Design review of the part built by this model. Coordinates are the model's own, in mm. A direction names the side the tool comes from. Round coordinates to 2 decimals unless told otherwise and drop trailing zeros. Order: outer loops, then holes, each group sorted by start corner. A loop starts at its lowest first (then second) coordinate and runs counter-clockwise, first axis right, second up. Notation, with made-up numbers: (69, -16.5) - (120, -16.5) arc R16 cw to (120, -0.5) - close; hole circle Ø6 at (67.25, 61). An arc over 180 degrees is marked (long way). Answer as a JSON object with one key per item and string values. Group by question number.
from build123d import *

# Parameters (mm, degrees)
F1_DEPTH = 50.8


with BuildPart() as f1:
    # F0 (on Front) → F1 (new body)
    with BuildSketch(Plane.XZ):
        with BuildLine():
            ThreePointArc((-7.481652, 37.285154), (-41.440481, 30.054075), (-70.981652, 11.811))
            Line((-70.981652, 11.811), (-20.181652, 11.811))
            ThreePointArc((-20.181652, 11.811), (-7.481652, 24.455001), (5.218348, 11.811))
            Line((5.218348, 11.811), (81.418348, 11.811))
            ThreePointArc((81.418348, 11.811), (94.118348, 24.369807), (106.818348, 11.811))
            Line((106.818348, 11.811), (157.618348, 11.811))
            ThreePointArc((157.618348, 11.811), (128.077177, 30.054075), (94.118348, 37.285154))
            ThreePointArc((94.118348, 37.285154), (43.318348, 50.896973), (-7.481652, 37.285154))
        make_face()
        with BuildLine():
            ThreePointArc((5.218348, 11.811), (-7.481652, 24.455001), (-20.181652, 11.811))
            ThreePointArc((-20.181652, 11.811), (-7.481652, -0.420556), (5.218348, 11.811))
        make_face()
        with BuildLine():
            ThreePointArc((106.818348, 11.811), (94.118348, 24.369807), (81.418348, 11.811))
            ThreePointArc((81.418348, 11.811), (94.118348, -1.27557), (106.818348, 11.811))
        make_face()
    extrude(amount=F1_DEPTH)


solid = f1.part
1. Tool access review of faces 1 (the flat face through (132, -25, 11.811)), 2 (the flat face through (43, -25, 11.811)), 3 (the flat face through (42, 0, 25)): name each direction out of +Z, -Z, +X, -X, +Y, -Y from which nothing blocks a thin tool from reaching the whole face with its end or side.
2. Take a section at C-C, the plane x = 36. Give the boundary of the cut face in (y, z), then the cut area to 3 significant figures.
3. Clearance check with flat-ended pins moving along their axes: P1, Ø2, axis at y = -10.5, z = 31, coming from the +X side; P2, Ø1, axis at y = -39, z = 21.5, coming from the +X side; P3, Ø2, axis at x = 19.5, y = -32.5, coming from the -Z side. State where each tip first meets the part, or that it passes through.
4. To check wall thickness, follow line 1 (X direction, y = -13.5, z = 11); line 2 (Z direction, x = -17, y = -17); line 3 (Z direction, x = -44.5, y = -7). State the ranges of each line that lie inside material, in increasing order. Write a range as from..to.
5. Take a section at D-D, the plane z = 46. Give the boundary of the cut face in (x, y).
6. Take a section at A-A, the plane z = 9. Give the boundary of the cut face in (x, y), then the cut area to 3 significant figures.
7. Take a section at B-B, the plane y = -9. Give the boundary of the cut face in (x, z), then the cut area to 3 significant figures.
8. Mouldability with a two-part tool opening along X and no side actions: class faces 4 (the cylindrical face through (44.063, -25.044, 50.894)), 5 (the cylindrical face through (93.834, -25.044, -1.272)), 6 (the flat face through (-46, -25, 11.811)) as pulls with the +X half, pulls with the -X half, needs draft (parallel to the pull), parting line crosses it, or undercut.
Response values:
{
 "1": {"face 1": "-Z, +X, +Y, -Y", "face 2": "-Z, +Y, -Y", "face 3": "+Z, -Z, +X, -X, +Y"},
 "2": {"outline": "(-50.8, 11.81) - (0, 11.81) - (0, 50.63) - (-50.8, 50.63) - close", "area": "1,970 mm2"},
 "3": {"P1": "x = 128.21", "P2": "x = 145.53", "P3": "z = 11.81"},
 "4": {"line 1": "-20.13..5.16, 81.42..106.82", "line 2": "3.87..36.47", "line 3": "11.81..28.77"},
 "5": {"outline": "(12.16, -50.8) - (74.48, -50.8) - (74.48, 0) - (12.16, 0) - close"},
 "6": {"outline": "(-19.76, -50.8) - (4.79, -50.8) - (4.79, 0) - (-19.76, 0) - close; (81.65, -50.8) - (106.59, -50.8) - (106.59, 0) - (81.65, 0) - close", "area": "2,510 mm2"},
 "7": {"outline": "(-70.98, 11.81) - (-20.18, 11.81) arc R12.71 ccw to (5.22, 11.81) - (81.42, 11.81) arc R12.71 ccw (long way) to (106.82, 11.81) - (157.62, 11.81) arc R101.6 ccw to (94.12, 37.29) arc R101.6 ccw to (-7.48, 37.29) arc R101.6 ccw to start", "area": "6,190 mm2"},
 "8": {"face 4": "parting line crosses it", "face 5": "undercut", "face 6": "needs draft"}
}
